Read the model definition and answer for the solid it produces. Units are mm, in the model's axes. A direction names the side the tool comes from. Coordinates: 2 decimals unless noted, no trailing zeros. Answer as a JSON object with one key per item and string values. Group by question number.
(1) Which of the six approach directions +Z, -Z, +X, -X, +Y, -Y give full straight-line access (tool end or side, diameter ignored) to faces 1 (the face through (-2, 1, 0)), 2 (the face through (-83, -22.225, 10))?
(2) Flat-ended cylindrical pins translate along their axes: P1, Ø7.5, axis at x = -83, z = 10, coming from the -Y side (3 decimals); P2, Ø4, axis at x = -55.5, y = -14.5, coming from the -Z side; P3, Ø1.6, axis at x = 101.5, y = 6, coming from the +Z side (3 decimals). Find the tip coordinate at first contact, or state that the pin passes through.
(3) Straight lines are drawn through the part: L1, parallel to X at y = 34, z = 17.75; L2, parallel to Z at x = 82, y = -36. For each, find the intervals that lie inside material, in ascending order.
(4) For a pull along Z with two mould halves and no side action, classify faces 3 (the face through (78.15, -31.88, 7.7)), 4 (the face through (106, 1, 19.05)), 5 (the face through (83, -22.225, 10)), 6 (the face through (-2, -41.275, 9)) as +Z half, -Z half, draft (parallel to the pull), parting line (faces both ways), or undercut.
from build123d import *

# Parameters (mm, degrees)
SKETCH1_W           = 215.9
SKETCH1_H           = 82.55
BOSS_EXTRUDE2_DEPTH = 19.05
SKETCH3_R           = 4.7625
CUT_EXTRUDE1_DEPTH  = 19.05
SKETCH5_W           = 3.175
SKETCH5_H           = 3.175
CUT_EXTRUDE2_DEPTH  = 83.55


with BuildPart() as part:
    # Sketch1 → Boss-Extrude2 (new body)
    with BuildSketch(Plane.XY):
        Rectangle(SKETCH1_W, SKETCH1_H)
    extrude(amount=BOSS_EXTRUDE2_DEPTH)

    # Sketch3 → Cut-Extrude1 (cut)
    with BuildSketch(Plane.XZ.offset(41.275)):
        with Locations((-82.55, 9.525)):
            Circle(SKETCH3_R)
    cut_extrude1 = extrude(amount=-CUT_EXTRUDE1_DEPTH, mode=Mode.SUBTRACT)

    # Sketch5 → Cut-Extrude2 (cut, through all)
    with BuildSketch(Plane.XZ.offset(41.275)):
        with Locations((-101.7905, 17.4625)):
            Rectangle(SKETCH5_W, SKETCH5_H)
    cut_extrude2 = extrude(amount=-CUT_EXTRUDE2_DEPTH, mode=Mode.SUBTRACT)

    # Mirror1: Cut-Extrude1, Cut-Extrude2 across plane
    add(cut_extrude1.mirror(Plane(origin=(0, 0, 0), x_dir=(0, 0, 1), z_dir=(1, 0, 0))), mode=Mode.SUBTRACT)
    add(cut_extrude2.mirror(Plane(origin=(0, 0, 0), x_dir=(0, 0, 1), z_dir=(1, 0, 0))), mode=Mode.SUBTRACT)


solid = part.part
Results below:
{
 "1": {"face 1": "-Z, +X, -X, +Y, -Y", "face 2": "-Y"},
 "2": {"P1": "stops at y = -22.225", "P2": "stops at z = 0", "P3": "stops at z = 15.875"},
 "3": {"L1": "x = -107.95 to -103.38, -100.2 to 100.2, 103.38 to 107.95", "L2": "z = 0 to 4.79, 14.26 to 19.05"},
 "4": {"face 3": "undercut", "face 4": "+Z half", "face 5": "undercut", "face 6": "draft"}
}
